For this review, use the dimensioned drawing (mm, ordinates from the lowest corner) and the shaded views. Coordinates: 2 decimals unless noted, no trailing zeros. Loops run counter-clockwise (first coordinate to the right, second up) from the corner with the lowest first, then second, coordinate; pieces in that order, holes last. Notation, with made-up numbers: M 16,85 L 31,85 A27 cw 31,101 Z; hole C 56,46 d8. An arc over 180 degrees is marked long. One line per item, written item: value.
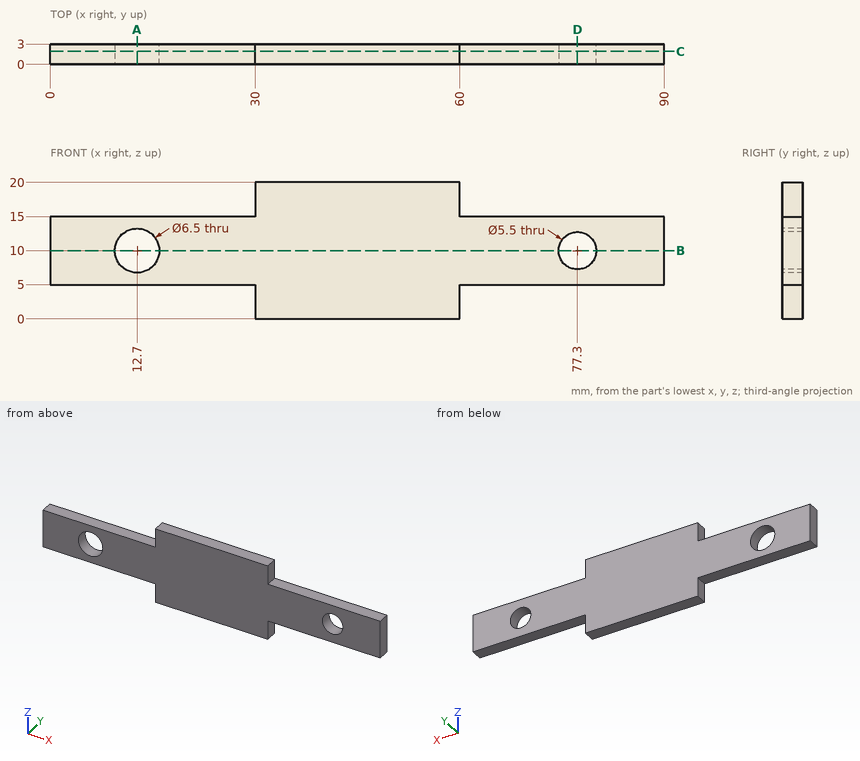
(1) We need section A-A on x = 12.7. State the section outline as (y, z) points, then the cut area to 3 significant figures.
Reply:
outline: M 0,5 L 3,5 L 3,6.75 L 0,6.75 Z; M 0,13.25 L 3,13.25 L 3,15 L 0,15 Z
area: 10.5 mm2
(2) Insertion check: pin 1 (1.5 mm diameter, centred on y = 1.5, z = 17.5, fed in from +X); pin 2 (1.5 mm diameter, centred on y = 1.5, z = 17, fed in from -X); pin 3 (1.5 mm diameter, centred on x = 76.5, y = 1.5, fed in from +Z). Each pin has a flat end and moves straight along its axis. Give the tip position at first contact, or say it passes through.
Reply:
pin 1: stops at x = 60
pin 2: stops at x = 30
pin 3: stops at z = 15
(3) We need section C-C on y = 1.9. State the section outline as (x, z) points, then the cut area to 3 significant figures.
Reply:
outline: M 0,5 L 30,5 L 30,0 L 60,0 L 60,5 L 90,5 L 90,15 L 60,15 L 60,20 L 30,20 L 30,15 L 0,15 Z; hole C 12.7,10 d6.5; hole C 77.3,10 d5.5
area: 1,140 mm2
(4) To check wall thickness, follow line 1 along X through (y, z) = (2.05, 10); line 2 along Z through (x, y) = (12.7, 0.9); line 3 along Z through (x, y) = (77.3, 2.05). State the ranges of each line that lie inside material, in increasing order. Write a range as [from, to].
Reply:
line 1: x = [0, 9.45], [15.95, 74.55], [80.05, 90]
line 2: z = [5, 6.75], [13.25, 15]
line 3: z = [5, 7.25], [12.75, 15]
(5) We need section D-D on x = 77.3. State the section outline as (y, z) points, then the cut area to 3 significant figures.
Reply:
outline: M 0,5 L 3,5 L 3,7.25 L 0,7.25 Z; M 0,12.75 L 3,12.75 L 3,15 L 0,15 Z
area: 13.5 mm2
(6) We need section B-B on z = 10. State the section outline as (x, y) points, then the cut area to 3 significant figures.
Reply:
outline: M 0,0 L 9.45,0 L 9.45,3 L 0,3 Z; M 15.95,0 L 74.55,0 L 74.55,3 L 15.95,3 Z; M 80.05,0 L 90,0 L 90,3 L 80.05,3 Z
area: 234 mm2
